The listing builds one solid part. Answer for the finished solid, in the listing's coordinates (mm). Face numbers are marked on the shaded views. Round coordinates to 2 decimals unless told otherwise and drop trailing zeros. Order: outer loops, then holes, each group sorted by start corner. A loop starts at its lowest first (then second) coordinate and runs counter-clockwise, first axis right, second up. Notation, with made-up numbers: (31, 39) -> (71, 39) arc R10 cw to (71, 56) -> close; hole circle Ø7 at (51, 79). An arc over 180 degrees is marked (long way). Answer in a Markdown table with one row per item. Add a question column.
Autodesk Inventor part; units mm, degrees
ref_plane "YZ Plane" through (0, 0, 0) normal (1, 0, 0) x (0, 1, 0)
ref_plane "XZ Plane" through (0, 0, 0) normal (0, 1, 0) x (-1, 0, 0)
ref_plane "XY Plane" through (0, 0, 0) normal (0, 0, 1) x (1, 0, 0)
sketch "Sketch1" plane through (0, 0, 0) normal (0, 1, 0) x (-1, 0, 0)
  line L0 (71.9808, 153.586) -> (11.2408, 153.586)
  line L1 (11.2408, 153.586) -> (11.2408, 50.288)
  line L2 (11.2408, 50.288) -> (71.9808, 50.288)
  line L3 (71.9808, 50.288) -> (71.9808, 153.586)
  point P0 (0, 0)
  dimension "d0" = 60.74
  dimension "d1" = 103.298
extrude "Extrusion1" add sketch "Sketch1" along normal blind 1
sketch "Sketch2" plane through (0, 1, 0) normal (0, 1, 0) x (1, 0, 0)
  line L0 (-71.9808, -50.288) -> (-71.9808, -153.586)
  line L1 (-11.2408, -153.586) -> (-11.2408, -50.288)
  line L2 (-71.9808, -153.586) -> (-11.2408, -153.586)
  line L3 (-11.2408, -153.586) -> (-11.2408, -151.586)
  line L4 (-11.2408, -151.586) -> (-71.9808, -151.586)
  line L5 (-71.9808, -151.586) -> (-71.9808, -153.586)
  line L6 (-11.2408, -50.288) -> (-71.9808, -50.288)
  line L7 (-71.9808, -151.586) -> (-70.9808, -151.586)
  line L8 (-70.9808, -151.586) -> (-70.9808, -50.288)
  line L9 (-70.9808, -50.288) -> (-71.9808, -50.288)
  line L10 (-71.9808, -50.288) -> (-71.9808, -151.586)
  line L11 (-70.9808, -50.288) -> (-11.2408, -50.288)
  line L12 (-11.2408, -50.288) -> (-11.2408, -52.288)
  line L13 (-11.2408, -52.288) -> (-70.9808, -52.288)
  line L14 (-70.9808, -52.288) -> (-70.9808, -50.288)
  line L15 (-11.2408, -52.288) -> (-12.2408, -52.288)
  line L16 (-12.2408, -52.288) -> (-12.2408, -151.586)
  line L17 (-12.2408, -151.586) -> (-11.2408, -151.586)
  line L18 (-11.2408, -151.586) -> (-11.2408, -52.288)
  point P0 (0, 0)
  dimension "d4" = 2
  dimension "d5" = 1
  dimension "d6" = 2
  dimension "d7" = 1
extrude "Extrusion2" add sketch "Sketch2" along normal blind 4.8 contours L6 L8 L4 L0 | L4 L1 L2 L0 | L6 L1 L13 L8 | L16 L13 L1 L4
sketch "Sketch3" plane through (0, 5.8, 0) normal (0, 1, 0) x (1, 0, 0)
  line L0 (-71.9808, -50.288) -> (-71.9808, -153.586)
  line L1 (-71.9808, -153.586) -> (-71.9808, -141.686)
  line L2 (-70.9808, -52.288) -> (-70.9808, -151.586)
  line L3 (-71.9808, -141.686) -> (-70.9808, -141.686)
  line L4 (-70.9808, -141.686) -> (-70.9808, -129.786)
  line L5 (-70.9808, -129.786) -> (-71.9808, -129.786)
  line L6 (-71.9808, -129.786) -> (-71.9808, -141.686)
  point P0 (0, 0)
  point P1 (-71.4808, -129.786)
  point P2 (-71.4808, -141.686)
  dimension "d18" = 11.9
  dimension "d19" = 11.9
extrude "Extrusion3" add sketch "Sketch3" along normal blind 5
sketch "Sketch4" plane through (0, 5.8, 0) normal (0, 1, 0) x (1, 0, 0)
  line L0 (-71.9808, -129.786) -> (-71.9808, -116.586)
  line L1 (-71.9808, -50.288) -> (-71.9808, -129.786)
  line L2 (-70.9808, -129.786) -> (-70.9808, -52.288)
  line L3 (-71.9808, -116.586) -> (-70.9808, -116.586)
  line L4 (-70.9808, -116.586) -> (-70.9808, -110.586)
  line L5 (-70.9808, -110.586) -> (-71.9808, -110.586)
  line L6 (-71.9808, -110.586) -> (-71.9808, -116.586)
  line L7 (-71.9808, -110.586) -> (-71.9808, -102.186)
  line L8 (-71.9808, -102.186) -> (-70.9808, -102.186)
  line L9 (-70.9808, -102.186) -> (-70.9808, -95.186)
  line L10 (-70.9808, -95.186) -> (-71.9808, -95.186)
  line L11 (-71.9808, -95.186) -> (-71.9808, -102.186)
  point P0 (0, 0)
  point P1 (-71.4808, -110.586)
  point P2 (-71.4808, -116.586)
  point P3 (-71.4808, -95.186)
  point P4 (-71.4808, -102.186)
  dimension "d22" = 13.2
  dimension "d23" = 6
  dimension "d24" = 8.4
  dimension "d25" = 7
extrude "Extrusion4" add sketch "Sketch4" along normal blind 2 contours L10 L2 L8 L1
sketch "Sketch5" plane through (0, 5.8, 0) normal (0, 1, 0) x (1, 0, 0)
  line L0 (-71.9808, -95.186) -> (-71.9808, -102.186)
  line L1 (-71.9808, -95.186) -> (-71.9808, -80.186)
  line L2 (-71.9808, -50.288) -> (-71.9808, -95.186)
  line L3 (-70.9808, -95.186) -> (-70.9808, -52.288)
  line L4 (-71.9808, -80.186) -> (-70.9808, -80.186)
  line L5 (-70.9808, -80.186) -> (-70.9808, -62.186)
  line L6 (-70.9808, -62.186) -> (-71.9808, -62.186)
  line L7 (-71.9808, -62.186) -> (-71.9808, -80.186)
  point P0 (0, 0)
  point P1 (-71.4808, -62.186)
  point P2 (-71.4808, -80.186)
  dimension "d28" = 15
  dimension "d29" = 18
extrude "Extrusion5" add sketch "Sketch5" along normal blind 3.9
sketch "Sketch6" plane through (0, 1, 0) normal (0, 1, 0) x (1, 0, 0)
  line L0 (-70.9808, -62.186) -> (-70.9808, -52.288)
  line L1 (-70.9808, -52.288) -> (-69.9808, -52.288)
  line L2 (-69.9808, -52.288) -> (-69.9808, -60.288)
  line L3 (-69.9808, -60.288) -> (-70.9808, -60.288)
  line L4 (-70.9808, -60.288) -> (-70.9808, -52.288)
  line L5 (-12.2408, -151.586) -> (-17.2408, -151.586)
  line L6 (-17.2408, -151.586) -> (-17.2408, -150.586)
  line L7 (-17.2408, -150.586) -> (-12.2408, -150.586)
  line L8 (-12.2408, -150.586) -> (-12.2408, -151.586)
  point P0 (0, 0)
  point P1 (-70.4808, -52.288)
  point P2 (-70.4808, -60.288)
  point P3 (-17.2408, -151.086)
  point P4 (-12.2408, -151.086)
  dimension "d32" = 1
  dimension "d33" = 8
  dimension "d34" = 1
  dimension "d35" = 5
extrude "Extrusion6" add sketch "Sketch6" along normal blind 10
properties part number "lid top"
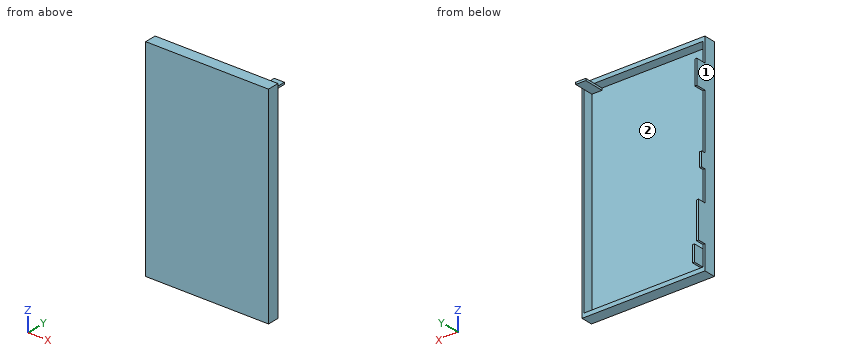
1. The mould has two halves that part along Z. Classify the marked faces 1 and 2: released by +Z, released by -Z, zero draft, split by the parting line, or undercut.
2. The part is cut by section A-A (x = -29.5). Give the vertices of the cut face in (y, z), then the cut area to 3 significant figures.
3. The part is cut by section C-C (y = 2.75). Give the vertices of the cut face in (x, z).
4. The part is cut by section D-D (x = -15.5). Give the vertices of the cut face in (y, z).
5. Each of these flat-tipped pins is pushed along its axis until it touches: pin 1 (1.1 mm diameter, centred on x = -71.5, z = 122.5, fed in from +Y); pin 2 (3 mm diameter, centred on x = -24.5, z = 99, fed in from -Y); pin 3 (3 mm diameter, centred on x = -42, z = 129, fed in from +Y); pin 4 (0.5 mm diameter, centred on x = -71.5, y = 7.5, fed in from +Z). Where does it stop, or does it pass through?
6. Straight lines are drawn through the part: line 1 along X through (y, z) = (3.5, 124.5); line 2 along Z through (x, y) = (-67.5, 5.75); line 3 along Y through (x, z) = (-64, 131). For each, find the intervals that lie inside material, in ascending order.
7. The part is cut by section B-B (z = 126). Give the vertices of the cut face in (x, y).
Report:
| question | item | result |
|---|---|---|
| 1 | face 1 | zero draft |
| 1 | face 2 | undercut |
| 2 | outline | (0, 50.29) -> (5.8, 50.29) -> (5.8, 52.29) -> (1, 52.29) -> (1, 151.59) -> (5.8, 151.59) -> (5.8, 153.59) -> (0, 153.59) -> close |
| 2 | area | 122 mm^2 |
| 3 | outline | (-71.98, 50.29) -> (-11.24, 50.29) -> (-11.24, 153.59) -> (-71.98, 153.59) -> close; hole (-70.98, 60.29) -> (-69.98, 60.29) -> (-69.98, 52.29) -> (-12.24, 52.29) -> (-12.24, 150.59) -> (-17.24, 150.59) -> (-17.24, 151.59) -> (-70.98, 151.59) -> close |
| 4 | outline | (0, 50.29) -> (5.8, 50.29) -> (5.8, 52.29) -> (1, 52.29) -> (1, 150.59) -> (11, 150.59) -> (11, 151.59) -> (5.8, 151.59) -> (5.8, 153.59) -> (0, 153.59) -> close |
| 5 | pin 1 | stops at y = 5.8 |
| 5 | pin 2 | stops at y = 0 |
| 5 | pin 3 | stops at y = 1 |
| 5 | pin 4 | stops at z = 141.69 |
| 6 | line 1 | x = -71.98 to -70.98, -12.24 to -11.24 |
| 6 | line 2 | z = 50.29 to 52.29, 151.59 to 153.59 |
| 6 | line 3 | y = 0 to 1 |
| 7 | outline | (-71.98, 0) -> (-11.24, 0) -> (-11.24, 5.8) -> (-12.24, 5.8) -> (-12.24, 1) -> (-70.98, 1) -> (-70.98, 5.8) -> (-71.98, 5.8) -> close |
